Autodesk Inventor part; units mm, degrees
ref_plane "YZ Plane" through (0, 0, 0) normal (1, 0, 0) x (0, 1, 0)
ref_plane "XZ Plane" through (0, 0, 0) normal (0, 1, 0) x (-1, 0, 0)
ref_plane "XY Plane" through (0, 0, 0) normal (0, 0, 1) x (1, 0, 0)
sketch "Esboço1" plane through (0, 0, 0) normal (0, 1, 0) x (-1, 0, 0)
  circle A0 centre (0, 0) radius 9
  dimension "d0" = 18
extrude "Extrusão1" add sketch "Esboço1" along normal blind 3
fillet "Arredondamento1" radius 2.5 1 edges at (9, 3, 0)
sketch "Esboço2" plane through (0, 0, 0) normal (1, 0, 0) x (0, 1, 0)
  line L0 (3, 6.5) -> (3, -6.5)
  line L1 (0, 0) -> (13.7463, 0)
  arc A0 (15, 0) -> (0, 0) centre (7.5, 0) ccw
  line L2 (0, 9) -> (0, -9)
  line L3 (15, 0) -> (0, 0)
  dimension "d4" = 15
revolve "Revolução1" add sketch "Esboço2" angle 360 about axis through (0, 0, 0) along (0, 1, 0)
fillet "Arredondamento2" radius 1 1 edges at (0, 3, -6)
hole "Furo1" at (0, 0, 0) direction (0, 1, 0) diameter 2.4 depth 8
properties part number "Puxador" material "Plástico PC/ABS"
Check sheet for the modelled part. Datum: model origin and axes. Units: mm. Coordinates: 2 decimals unless noted, no trailing zeros. Order: outer loops, then holes, each group sorted by start corner. A loop starts at its lowest first (then second) coordinate and runs counter-clockwise, first axis right, second up. Notation, with made-up numbers: (17, -17) -> (51, -17) arc R23 cw to (51, 4) -> close; hole circle Ø10 at (-16, 72.25). An arc over 180 degrees is marked (long way). Write each question's results on one line, items separated by ' | '. Start each with the question number.
1) Material ranges on line 1 along X through (y, z) = (2, 0); line 2 along Z through (x, y) = (0, 4); line 3 along X through (y, z) = (2.5, 0), recorded low to high.
2) Section check B-B (y = 12). Enter the section's corners in (x, z), and give its area (3 significant figures).
3) Depth check by flat-ended pin: pin 1 (1.5 mm diameter, centred on x = -1, y = 6, fed in from +Z); pin 2 (2 mm diameter, centred on x = 4.5, y = 7.5, fed in from -Z); pin 3 (4 mm diameter, centred on x = 6, z = -5.5, fed in from -Y); pin 4 (1.5 mm diameter, centred on x = 4, y = 12.5, fed in from +Z). Enter the tip coordinate at first touch or a pass-through.
4) Section check C-C (y = 5). Enter the section's corners in (x, z).
5) Draft check along X on faces 1 (the face through (1.172, 0.246, -8.923)), 2 (the face through (-1.01, 4.06, -0.65)), 3 (the face through (0, 0, -2)). Enter one of: pulls with the +X half, pulls with the -X half, needs draft (parallel to the pull), parting line crosses it, or undercut.
6) Section check A-A (y = 2). Enter the section's corners in (x, z), and give its area (3 significant figures).
Checked values:
1) line 1: -8.5 to -1.2, 1.2 to 8.5 | line 2: -6.67 to -1.2, 1.2 to 6.67 | line 3: -8 to -1.2, 1.2 to 8
2) outline: circle Ø12 at (0, 0) | area: 113 mm²
3) pin 1: z = 7.43 | pin 2: z = -6.63 | pin 3: y = 0 | pin 4: z = 4.93
4) outline: circle Ø14.14 at (0, 0); hole circle Ø2.4 at (0, 0)
5) face 1: parting line crosses it | face 2: undercut | face 3: needs draft
6) outline: circle Ø17 at (0, 0); hole circle Ø2.4 at (0, 0) | area: 222 mm²
